Source: CAD feature listing. Evaluate the final solid. Frame: model axes, mm. Face numbers are marked on the shaded views. A direction names the side the tool comes from. Coordinates: 2 decimals unless noted, no trailing zeros. Write each loop counter-clockwise with the first axis right and the second up, starting at its lowest first coordinate (ties: lowest second). Pieces come first, ordered by that corner, then holes. Notation, with made-up numbers: M -32,47 L 26,47 A22 ccw 26,83 Z; hole C 79.25,72 d1. An arc over 180 degrees is marked long. Write item = value, one per line. Start each with the question number.
1. Section query D-D (x = -5). Output: boundary loops of the cut face in (y, z).
2. Section query B-B (y = 0). Output: boundary loops of the cut face in (x, z), then the cut area to 3 significant figures.
3. Section query C-C (x = -11.5). Output: boundary loops of the cut face in (y, z).
4. Access query for the marked faces 4, 5, 6 and 7. Directions: +Z, -Z, +X, -X, +Y, -Y. A direction counts if a zero-diameter tool reaches every point of the face in a straight line with its end or side. Return the directions, or none.
5. Section query A-A (z = 5). Output: boundary loops of the cut face in (x, y).
6. Pin query (flat end, axial travel): pin 1 Ø3.5 at (y, z) = (-35, 5) entering from +X; pin 2 Ø5 at (y, z) = (-44.5, 5) entering from -X; pin 3 Ø5 at (y, z) = (-32, 5) entering from +X; pin 4 Ø4.5 at (y, z) = (-35, 5) entering from -X. Return the tip coordinate at first contact, or that it passes through.
7. Line query: line 1 along Y through (x, z) = (4.5, 3.75); line 2 along X through (y, z) = (-35.5, 9.25); line 3 along Z through (x, y) = (5, -35). Output: solid intervals per line, ascending.
8. Pull-direction query (X, two-part tool) for the marked faces 1, 2 and 3; classes: pulls with the +X half, pulls with the -X half, needs draft (parallel to the pull), parting line crosses it, or undercut.
```python
from build123d import *

# Parameters (mm, degrees)
F1_DEPTH = 10
F3_DEPTH = 25
F4_R     = 2.6
F5_DEPTH = 25


with BuildPart() as f1:
    # F0 (on Top) → F1 (new body)
    with BuildSketch(Plane.XY):
        with BuildLine():
            ThreePointArc((-2, -25.922963), (0, 26), (2, -25.922963))
            Line((2, -25.922963), (2, -40))
            Line((2, -40), (8, -40))
            Line((8, -40), (8, -35.721142))
            ThreePointArc((8, -35.721142), (9.485307, -30.477098), (13.5, -26.790857))
            ThreePointArc((13.5, -26.790857), (0, 30), (-13.5, -26.790857))
            ThreePointArc((-13.5, -26.790857), (-9.485307, -30.477098), (-8, -35.721142))
            Line((-8, -35.721142), (-8, -50))
            Line((-8, -50), (-2, -50))
            Line((-2, -50), (-2, -25.922963))
        make_face()
    extrude(amount=F1_DEPTH)

    # F2 (on Right) → F3 (cut)
    with BuildSketch(Plane.YZ):
        with BuildLine():
            ThreePointArc((-37.1, 5), (-35, 2.9), (-32.9, 5))
            ThreePointArc((-32.9, 5), (-35, 7.1), (-37.1, 5))
        make_face()
    extrude(amount=-F3_DEPTH, mode=Mode.SUBTRACT)

    # F4 (on Right) → F5 (cut)
    with BuildSketch(Plane.YZ):
        with Locations((-35, 5)):
            Circle(F4_R)
    extrude(amount=F5_DEPTH, mode=Mode.SUBTRACT)


solid = f1.part
```
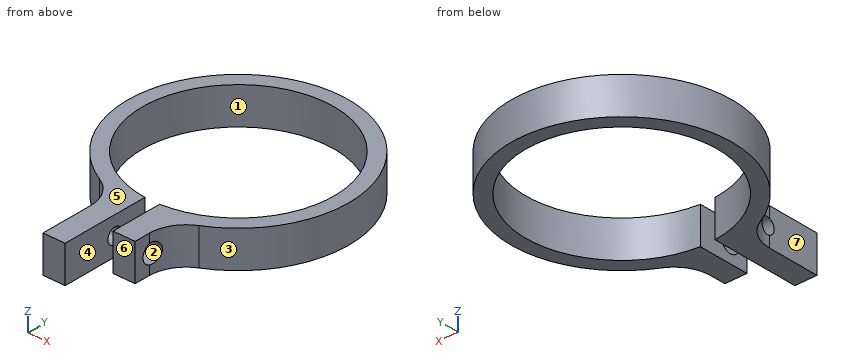
Results are:
q1.outline = M -50,0 L -25.51,0 L -25.51,10 L -50,10 Z; M 25.51,0 L 29.58,0 L 29.58,10 L 25.51,10 Z; hole C -35,5 d4.2
q2.outline = M -30,0 L -26,0 L -26,10 L -30,10 Z; M 26,0 L 30,0 L 30,10 L 26,10 Z
q2.area = 80.0 mm^2
q3.outline = M -28.12,0 L -23.32,0 L -23.32,10 L -28.12,10 Z; M 23.32,0 L 27.71,0 L 27.71,10 L 23.32,10 Z
q4.face_4 = +Z, -Z, -Y
q4.face_5 = +Z, +X, -X, +Y, -Y
q4.face_6 = +Z, -Z, +X, -Y
q4.face_7 = +Z, -Z, -X, -Y
q5.outline = M -13.5,-26.79 A10 cw -8.41,-32.9 L -2,-32.9 L -2,-25.92 A26 cw long 2,-25.92 L 2,-32.4 L 8.57,-32.4 A10 cw 13.5,-26.79 A30 ccw long Z; M -8,-50 L -2,-50 L -2,-37.1 L -8,-37.1 Z; M 2,-40 L 8,-40 L 8,-37.6 L 2,-37.6 Z
q6.pin_1 = through
q6.pin_2 = -8
q6.pin_3 = 10.17
q6.pin_4 = -8.45
q7.line_1 = -40 to -37.28, -32.72 to -25.61, 25.61 to 29.66
q7.line_2 = -8 to -2, 2 to 8
q7.line_3 = 0 to 2.4, 7.6 to 10
q8.face_1 = undercut
q8.face_2 = needs draft
q8.face_3 = parting line crosses it
